from build123d import *

# Parameters (mm, degrees)
F1_DEPTH = 2.25
F0_W     = 41.148
F0_H     = 33.0774
F2_DEPTH = 15
F5_DEPTH = 50
F7_DEPTH = 11.5201335364
F8_DEPTH = 1.5
F9_R     = 1


with BuildPart() as f1:
    # F0 (on Front) → F1 (new body)
    with BuildSketch(Plane.XZ):
        Polygon((13.589, 17.5387), (13.589, 19.5707), (4.953, 19.5707), (4.953, 17.5387), (-4.953, 17.5387), (-4.953, 19.5707), (-13.589, 19.5707), (-13.589, 17.5387), (-20.574, 17.5387), (-20.574, 16.5387), (20.574, 16.5387), (20.574, 17.5387), align=None)
    extrude(amount=F1_DEPTH)


with BuildPart() as f1b:
    # F0 (on Front) → F1, piece 2 (new body)
    with BuildSketch(Plane.XZ):
        Polygon((20.574, -17.5387), (20.574, -16.5387), (-20.574, -16.5387), (-20.574, -17.5387), (-13.589, -17.5387), (-13.589, -19.5707), (-4.953, -19.5707), (-4.953, -17.5387), (4.953, -17.5387), (4.953, -19.5707), (13.589, -19.5707), (13.589, -17.5387), align=None)
    extrude(amount=F1_DEPTH)


with BuildPart() as f2:
    # F0 (on Front) → F2 (new body)
    with BuildSketch(Plane.XZ):
        Rectangle(F0_W, F0_H)
    extrude(amount=F2_DEPTH)


with BuildPart() as f1_1:
    add(f1.part)

    # F3: union F1b, F2
    add(f1b.part)
    add(f2.part)

    # F4 (on face) → F5 (cut)
    with BuildSketch(Plane.YZ.offset(20.574)):
        Polygon((-15, -16.5387), (-2.25, -16.5387), (-11.1130626177, 16.5387), (-15, 16.5387), align=None)
    extrude(amount=-F5_DEPTH, mode=Mode.SUBTRACT)

    # F6 (on face) → F7 (cut, through all)
    with BuildSketch(Plane(origin=(0, -6.2339535793, -1.6703828272), x_dir=(1, 0, 0), z_dir=(0, -0.9659258263, -0.2588190451))):
        with BuildLine():
            ThreePointArc((9, 3.8514297181), (6.3639610307, 10.2153907488), (0, 12.8514297181))
            ThreePointArc((0, 12.8514297181), (-6.3639610307, -2.5125313125), (9, 3.8514297181))
        make_face()
    extrude(amount=-F7_DEPTH, mode=Mode.SUBTRACT)

    # F6 (on face) → F8 (cut)
    with BuildSketch(Plane(origin=(0, -6.2339535793, -1.6703828272), x_dir=(1, 0, 0), z_dir=(0, -0.9659258263, -0.2588190451))):
        Polygon((11.1, 14.9514297181), (0, 14.9514297181), (-11.1, 14.9514297181), (-11.1, -7.2485702819), (11.1, -7.2485702819), align=None)
        with BuildLine():
            ThreePointArc((9, 3.8514297181), (-6.3639610307, -2.5125313125), (0, 12.8514297181))
            ThreePointArc((0, 12.8514297181), (6.3639610307, 10.2153907488), (9, 3.8514297181))
        make_face(mode=Mode.SUBTRACT)
    extrude(amount=-F8_DEPTH, mode=Mode.SUBTRACT)

    # F9
    f9_edges = [f1_1.edges().sort_by_distance(p)[0] for p in [
        (-9, 0, 3.987295),
        (-9, -5.781888, 2.438041),
    ]]
    fillet(f9_edges, radius=F9_R)


solid = f1_1.part
Design review of the part built by this model. Coordinates are the model's own, in mm. A direction names the side the tool comes from. Give positions to 0.01 mm unless a question says otherwise; leave off trailing zeros. Order: outer loops, then holes, each group sorted by start corner. A loop starts at its lowest first (then second) coordinate and runs counter-clockwise, first axis right, second up. Notation, with made-up numbers: (33, 72.25) - (37, 72.25) arc R17 ccw to (37, 103.25) - close; hole circle Ø8 at (66, -16). An arc over 180 degrees is marked (long way). Use CSV: the item, a comma, the result in double quotes. Start each with the question number.
Q1. Draft analysis for pull direction X (two halves, no side actions). For faces 1 (the face through (4.953, -1, 19)), 2 (the face through (-9, -1, 19.571)), 3 (the face through (20.574, -4, 4)), state which applies: pulls with the +X half, pulls with the -X half, needs draft (parallel to the pull), parting line crosses it, or undercut.
Q2. For line 1 (Z direction, x = -7, y = -2); line 2 (Y direction, x = -16.5, z = -17); line 3 (X direction, y = -2.75, z = 10), list the stretches that pass through material, from the lowest coordinate up.
Q3. Machinability: for faces 4 (the face through (-17, -1, -17.539)), 5 (the face through (0.155, -9.389, 12.963)), 6 (the face through (13.589, -1, -19)), which of the approach directions +Z, -Z, +X, -X, +Y, -Y give a long, thin tool a straight path to every point of the face, cutting with its end or side? Answer none if there is none.
Q4. For P1, Ø10, axis at x = 12.5, z = -10.5, coming from the -Y side; P2, Ø1.5, axis at x = 16, y = -1.5, coming from the -Z side; P3, Ø1.6, axis at y = -1.5, z = 19, coming from the +X side, all flat-tipped, find the tip position at first contact; note any pin that passes through.
Q5. Take a section at B-B (z = -10.5). State the section outline as (x, y) points.
Q6. Take a section at D-D (z = 15.5). State the section outline as (x, y) points, and give its area (3 significant figures).
Q7. Take a section at A-A (x = -10.5). State the section outline as (y, z) points, and give its area (3 significant figures).
Q8. Take a section at C-C (x = -16.5). State the section outline as (y, z) points, and give its area (3 significant figures).
Calculated:
1,face 1,"undercut"
1,face 2,"needs draft"
1,face 3,"pulls with the +X half"
2,line 1,"z = -19.57 to -2.41, 9.31 to 19.57"
2,line 2,"y = -2.25 to 0"
2,line 3,"x = -20.57 to -6.2, 6.2 to 20.57"
3,face 4,"-Z, -X, +Y, -Y"
3,face 5,"-Z"
3,face 6,"-Z, +X, +Y, -Y"
4,P1,"stops at y = -5.21"
4,P2,"stops at z = -17.54"
4,P3,"stops at x = 13.59"
5,outline,"(-20.57, -3.87) - (20.57, -3.87) - (20.57, 0) - (-20.57, 0) - close"
6,outline,"(-20.57, -10.83) - (20.57, -10.83) - (20.57, 0) - (-20.57, 0) - close"
6,area,"446 mm²"
7,outline,"(-11.11, 16.54) - (-10.1, 12.77) - (-8.65, 13.16) - (-2.91, -8.28) - (-4.36, -8.67) - (-2.25, -16.54) - (-2.25, -19.57) - (0, -19.57) - (0, 19.57) - (-2.25, 19.57) - (-2.25, 16.54) - close"
7,area,"201 mm²"
8,outline,"(-11.11, 16.54) - (-2.25, -16.54) - (-2.25, -17.54) - (0, -17.54) - (0, 17.54) - (-2.25, 17.54) - (-2.25, 16.54) - close"
8,area,"226 mm²"
